from build123d import *

# Parameters (mm, degrees)
SKETCH1_W           = 22.225
SKETCH1_H           = 22.225
BASE_EXTRUDE_DEPTH  = 12.7
FILLET1_R           = 1.5875
BOSS_EXTRUDE1_DEPTH = 49.2125
FILLET2_R           = 3.175
SHELL1_START        = 15.875
SHELL1_DEPTH        = 46.0375
SHELL1_2_OUTLINE_W  = 15.875
SHELL1_2_OUTLINE_H  = 15.875
SHELL1_2_DEPTH      = 15.875
FILLET4_R           = 1.5875


# Read off the part's stored shape, not the designer's step: Shell1
with BuildPart() as part:
    # Sketch1 → Base-Extrude (new body)
    with BuildSketch(Plane.XY):
        Rectangle(SKETCH1_W, SKETCH1_H)
    extrude(amount=BASE_EXTRUDE_DEPTH)

    # Fillet1
    fillet1_edges = [part.edges().sort_by_distance(p)[0] for p in [
        (-11.1125, 11.1125, 6.35),
        (11.1125, 11.1125, 6.35),
        (11.1125, -11.1125, 6.35),
        (-11.1125, -11.1125, 6.35),
    ]]
    fillet(fillet1_edges, radius=FILLET1_R)

    # Sketch2 → Boss-Extrude1 (add)
    with BuildSketch(Plane.XY.offset(12.7)):
        with BuildLine():
            Line((23.8125, -9.525), (23.8125, 9.525))
            ThreePointArc((23.8125, 9.525), (19.627788136, 19.627788136), (9.525, 23.8125))
            Line((9.525, 23.8125), (-9.525, 23.8125))
            ThreePointArc((-9.525, 23.8125), (-19.627788136, 19.627788136), (-23.8125, 9.525))
            Line((-23.8125, 9.525), (-23.8125, -9.525))
            ThreePointArc((-23.8125, -9.525), (-19.627788136, -19.627788136), (-9.525, -23.8125))
            Line((-9.525, -23.8125), (9.525, -23.8125))
            ThreePointArc((9.525, -23.8125), (19.627788136, -19.627788136), (23.8125, -9.525))
        make_face()
    extrude(amount=BOSS_EXTRUDE1_DEPTH)

    # Fillet2
    fillet2_edges = [part.edges().sort_by_distance(p)[0] for p in [
        (19.627788136, -19.627788136, 12.7),
        (23.8125, 0, 12.7),
        (19.627788136, 19.627788136, 12.7),
        (0, 23.8125, 12.7),
        (-19.627788136, 19.627788136, 12.7),
        (-23.8125, 0, 12.7),
        (-19.627788136, -19.627788136, 12.7),
        (0, -23.8125, 12.7),
    ]]
    fillet(fillet2_edges, radius=FILLET2_R)

    # Shell1 outline → Shell1 (cut)
    with BuildSketch(Plane.XY.offset(SHELL1_START)):
        with BuildLine():
            ThreePointArc((9.525, -20.6375), (17.382724106, -17.382724106), (20.6375, -9.525))
            Line((20.6375, -9.525), (20.6375, 9.525))
            ThreePointArc((20.6375, 9.525), (17.382724106, 17.382724106), (9.525, 20.6375))
            Line((9.525, 20.6375), (-9.525, 20.6375))
            ThreePointArc((-9.525, 20.6375), (-17.382724106, 17.382724106), (-20.6375, 9.525))
            Line((-20.6375, 9.525), (-20.6375, -9.525))
            ThreePointArc((-20.6375, -9.525), (-17.382724106, -17.382724106), (-9.525, -20.6375))
            Line((-9.525, -20.6375), (9.525, -20.6375))
        make_face()
    extrude(amount=SHELL1_DEPTH, mode=Mode.SUBTRACT)

    # Shell1 2 outline → Shell1 2 (cut)
    with BuildSketch(Plane.XY):
        Rectangle(SHELL1_2_OUTLINE_W, SHELL1_2_OUTLINE_H)
    extrude(amount=SHELL1_2_DEPTH, mode=Mode.SUBTRACT)

    # Fillet4
    fillet4_edges = [part.edges().sort_by_distance(p)[0] for p in [
        (0, -7.9375, 15.875),
        (0, 7.9375, 15.875),
        (-7.9375, 0, 15.875),
        (7.9375, 0, 15.875),
    ]]
    fillet(fillet4_edges, radius=FILLET4_R)


solid = part.part
Part model, mm, in its own coordinate system. A direction names the side the tool comes from. Give positions to 0.01 mm unless a question says otherwise; leave off trailing zeros. Loops run counter-clockwise (first coordinate to the right, second up) from the corner with the lowest first, then second, coordinate; pieces in that order, holes last.
(1) Drill centre lines: line 1 along X through (y, z) = (-0.5, 30.5); line 2 along Z through (x, y) = (11, 5.5) (3 decimals). Where is each one in solid material? Low to high.
Return value:
line 1: x = -23.81 to -20.64, 20.64 to 23.81
line 2: z = 0 to 15.875
(2) Band-saw the part on A-A (z = 10). Write the cut outline in (x, y) (1 decimal).
Return value:
outline: (-11.1, -9.5) arc R1.6 ccw to (-9.5, -11.1) - (9.5, -11.1) arc R1.6 ccw to (11.1, -9.5) - (11.1, 9.5) arc R1.6 ccw to (9.5, 11.1) - (-9.5, 11.1) arc R1.6 ccw to (-11.1, 9.5) - close; hole (-7.9, -7.9) - (7.9, -7.9) - (7.9, 7.9) - (-7.9, 7.9) - close
(3) Pull direction X, two halves, no side cores. Call faces 5 (the flat face through (0, -23.812, 39)), 6 (the cylindrical face through (19.516, -19.738, 38.571)), 7 (the cylindrical face through (8.41, 0.13, 15.42)): pulls with the +X half, pulls with the -X half, needs draft (parallel to the pull), parting line crosses it, or undercut.
Return value:
face 5: needs draft
face 6: pulls with the +X half
face 7: undercut
(4) 3-axis set-ups, long thin cutter, end or side, ignore diameter. For faces 1 (the flat face through (0, -11.112, 6)), 2 (the flat face through (0, 20.638, 39)), 3 (the flat face through (-7.938, 0, 7)), 4 (the cylindrical face through (10.66, 10.635, 6.439)): which of +Z, -Z, +X, -X, +Y, -Y reach the whole face in a straight line?
Return value:
face 1: -Z, +X, -X, -Y
face 2: +Z
face 3: +Z, -Z
face 4: -Z, +X, +Y
(5) Band-saw the part on D-D (z = 21). Write the cut outline in (x, y) (1 decimal).
Return value:
outline: (-23.8, -9.5) arc R14.3 ccw to (-9.5, -23.8) - (9.5, -23.8) arc R14.3 ccw to (23.8, -9.5) - (23.8, 9.5) arc R14.3 ccw to (9.5, 23.8) - (-9.5, 23.8) arc R14.3 ccw to (-23.8, 9.5) - close; hole (-20.6, -9.5) arc R11.1 ccw to (-9.5, -20.6) - (9.5, -20.6) arc R11.1 ccw to (20.6, -9.5) - (20.6, 9.5) arc R11.1 ccw to (9.5, 20.6) - (-9.5, 20.6) arc R11.1 ccw to (-20.6, 9.5) - close
(6) Pin check, flat tips, straight feed: pin 1 (14 mm diameter, centred on y = -4, z = 5, fed in from +X); pin 2 (6.5 mm diameter, centred on x = -3.5, z = 5, fed in from +Y); pin 3 (1.5 mm diameter, centred on x = -18, z = 27, fed in from +Y). Stop position of each tip, or through.
Return value:
pin 1: stops at x = 11.11
pin 2: stops at y = 11.11
pin 3: stops at y = 21.54
